Geometry: final body of the model. Coordinates: model frame, mm. Coordinates: 2 decimals unless noted, no trailing zeros. Write each loop counter-clockwise with the first axis right and the second up, starting at its lowest first coordinate (ties: lowest second). Pieces come first, ordered by that corner, then holes. Notation, with made-up numbers: (-34.75, 54.5) - (-20.75, 54.5) arc R22 ccw to (-20.75, 82.5) - close; hole circle Ø10 at (-21.75, 86). An arc over 180 degrees is marked (long way). Answer as a JSON object with one key per item and string values. Group by question number.
Item 1: Section A-A on z = 0. Return loops of the section in (x, y), and give its area (3 significant figures).
Item 2: Section B-B on x = 3.25. Return loops of the section in (y, z).
Item 3: Line query: line 1 along X through (y, z) = (-0.9, 1.25); line 2 along Z through (x, y) = (0.75, -0.4); line 3 along Z through (x, y) = (-5.75, -0.7). Output: solid intervals per line, ascending. Write a range as from..to.
Item 4: First-contact query: pin 1 Ø2.5 at (x, z) = (0.77, 2.38) entering from -Y; pin 2 Ø1.9 at (x, z) = (0.77, -2.38) entering from +Y. Flat tips, straight axial feed; report the tip coordinate or a pass-through.
Item 5: Section D-D on x = -4.25. Return loops of the section in (y, z).
Item 6: Section C-C on y = -0.85. State how many separate pieces and enclosed holes the cut face has, and give its area (3 significant figures).
```python
from build123d import *

# Parameters (mm, degrees)
F0_R     = 9
F1_DEPTH = 1
F3_D     = 2.0574
F3_DEPTH = 15
F3_TIP   = 0.6181053188


# Not quite as in the source:
# - a feature names something its author has since deleted; it is built from what else it names


with BuildPart() as f1:
    # F0 (on Front) → F1 (new body)
    with BuildSketch(Plane.XZ):
        Circle(F0_R)
    extrude(amount=F1_DEPTH)

    # F3
    with Locations(Plane.XZ.offset(1)):
        with Locations((-3.5267115138, 4.8541019662), (-5.7063390978, 1.8541019662), (-5.7063390978, -1.8541019662), (-3.5267115138, -4.8541019662), (0, -6), (3.5267115138, -4.8541019662), (5.7063390978, -1.8541019662), (0, 6), (-2.0225424859, 1.4694631307), (-2.0225424859, -1.4694631307), (0.7725424859, -2.3776412907), (2.5, 0), (0.7725424859, 2.3776412907), (3.5267115138, 4.8541019662), (5.7063390978, 1.8541019662)):
            Hole(F3_D / 2, depth=F3_DEPTH)
            with Locations((0, 0, -(F3_DEPTH + F3_TIP / 2))):  # 118° drill point
                Cone(0, F3_D / 2, F3_TIP, mode=Mode.SUBTRACT)


solid = f1.part
```
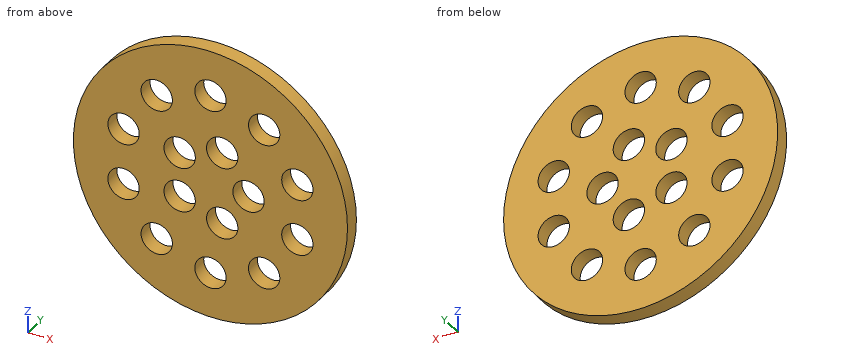
Checks:
{
 "1": {"outline": "(-9, -1) - (1.47, -1) - (1.47, 0) - (-9, 0) - close; (3.53, -1) - (9, -1) - (9, 0) - (3.53, 0) - close", "area": "15.9 mm^2"},
 "2": {"outline": "(-1, -8.39) - (0, -8.39) - (0, -5.84) - (-1, -5.84) - close; (-1, -3.86) - (0, -3.86) - (0, -0.7) - (-1, -0.7) - close; (-1, 0.7) - (0, 0.7) - (0, 3.86) - (-1, 3.86) - close; (-1, 5.84) - (0, 5.84) - (0, 8.39) - (-1, 8.39) - close"},
 "3": {"line 1": "-8.91..-6.54, -4.87..-3.03, -1.02..4.87, 6.54..8.91", "line 2": "-8.97..-6.7, -5.3..-3.41, -1.35..1.35, 3.41..5.3, 6.7..8.97", "line 3": "-6.92..-2.88, -0.83..0.83, 2.88..6.92"},
 "4": {"pin 1": "y = -1", "pin 2": "through"},
 "5": {"outline": "(-1, -7.93) - (0, -7.93) - (0, -5.59) - (-1, -5.59) - close; (-1, -4.12) - (0, -4.12) - (0, 4.12) - (-1, 4.12) - close; (-1, 5.59) - (0, 5.59) - (0, 7.93) - (-1, 7.93) - close"},
 "6": {"separate pieces": "1", "enclosed holes": "15", "area": "205 mm^2"}
}
